Autodesk Inventor part; units mm, degrees
ref_plane "YZ Plane" through (0, 0, 0) normal (1, 0, 0) x (0, 1, 0)
ref_plane "XZ Plane" through (0, 0, 0) normal (0, 1, 0) x (-1, 0, 0)
ref_plane "XY Plane" through (0, 0, 0) normal (0, 0, 1) x (1, 0, 0)
sketch "スケッチ1" plane through (0, 0, 0) normal (0, 0, 1) x (1, 0, 0)
  line L0 (0, 31) -> (26, 31)
  line L1 (26, 31) -> (26, 0)
  line L2 (26, 0) -> (0, 0)
  line L3 (0, 0) -> (0, 31)
  circle A0 centre (13, 31) radius 27.5
  point P0 (26, 6.7668)
  point P1 (0, 6.7668)
  dimension "d0" = 55
  dimension "d1" = 31
  dimension "d3" = 26
extrude "押し出し1" add sketch "スケッチ1" along normal blind 30 contours A0 L1 L2 L3
sketch "スケッチ2" plane through (0, 0, 0) normal (0, -1, 0) x (1, 0, 0)
  line L0 (26, 0) -> (0, 30)
  line L1 (0, 0) -> (26, 30)
  line L2 (22, 4.6154) -> (4, 4.6154)
  line L3 (4, 4.6154) -> (4, 25.3846)
  line L4 (4, 25.3846) -> (22, 25.3846)
  line L5 (22, 25.3846) -> (22, 4.6154)
  line L6 (26, 0) -> (26, 30)
  line L7 (26, 0) -> (0, 0)
  line L8 (0, 0) -> (0, 32)
  circle A0 centre (22, 4.6154) radius 0.8
  circle A1 centre (4, 4.6154) radius 0.8
  circle A2 centre (4, 25.3846) radius 0.8
  circle A3 centre (22, 25.3846) radius 0.8
  dimension "d6" = 4
  dimension "d7" = 1.6
  dimension "d8" = 1.6
  dimension "d9" = 1.6
  dimension "d10" = 1.6
extrude "押し出し2" cut sketch "スケッチ2" against normal through all contours A0 L2 L0 | L0 L5 A0 | L2 A0 L0 | L0 A0 L5 | A3 L5 L1 | L1 L4 A3 | A1 L3 L1 | L1 L2 A1 | L2 L1 A1 | L5 A3 L1 | L1 A3 L4 | L3 A1 L1 | A2 L4 L0 | L0 L3 A2 | A2 L0 L4 | L3 L0 A2
properties part number "toe_back_buf"
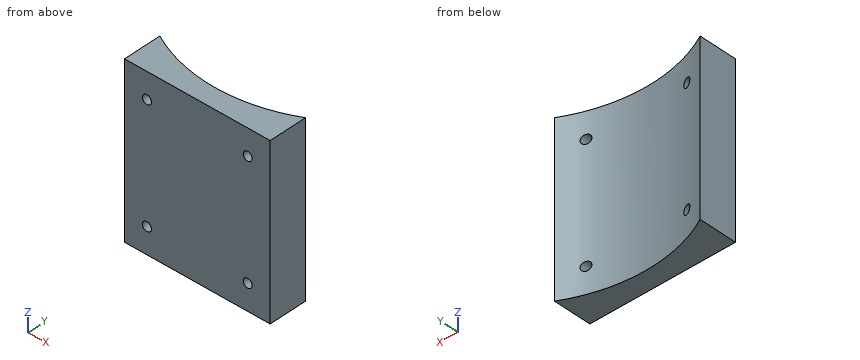
Geometry: final body of the model. Coordinates: model frame, mm. Round coordinates to 2 decimals unless told otherwise and drop trailing zeros. Order: outer loops, then holes, each group sorted by start corner. A loop starts at its lowest first (then second) coordinate and runs counter-clockwise, first axis right, second up. Notation, with made-up numbers: (-4, 58.5) - (33, 58.5) arc R10 cw to (33, 76.5) - close; hole circle Ø2 at (76.5, -19). An arc over 180 degrees is marked (long way). Write each question's results on one line, items separated by ' | '.
Item 1: Material intervals for line 1 along Z through (x, y) = (4, 4.05); line 2 along X through (y, z) = (2, 25); line 3 along X through (y, z) = (1.25, 4), sorted ascending. Write a range as [from, to].
Completed:
line 1: [0, 3.82], [5.42, 24.58], [26.18, 30] | line 2: [0, 3.3], [4.7, 21.3], [22.7, 26] | line 3: [0, 3.49], [4.51, 21.49], [22.51, 26]
Item 2: Section D-D, the plane x = 7.25. Return the cut outline in (y, z).
Completed:
outline: (0, 0) - (4.11, 0) - (4.11, 30) - (0, 30) - close
Item 3: Section B-B, the plane x = 4. Return the cut outline in (y, z), and give its area (3 significant figures).
Completed:
outline: (0, 0) - (5.01, 0) - (5.01, 3.82) - (0, 3.82) - close; (0, 5.42) - (5.01, 5.42) - (5.01, 24.58) - (0, 24.58) - close; (0, 26.18) - (5.01, 26.18) - (5.01, 30) - (0, 30) - close | area: 134 mm^2
Item 4: Section A-A, the plane y = 4. Return the cut outline in (x, z).
Completed:
outline: (0, 0) - (7.78, 0) - (7.78, 30) - (0, 30) - close; (18.22, 0) - (26, 0) - (26, 30) - (18.22, 30) - close; hole circle Ø1.6 at (4, 4.62); hole circle Ø1.6 at (4, 25.38); hole circle Ø1.6 at (22, 4.62); hole circle Ø1.6 at (22, 25.38)
Item 5: First-contact query: pin 1 Ø2 at (x, z) = (4, 25.38) entering from +Y; pin 2 Ø1.4 at (x, z) = (22, 4.62) entering from +Y; pin 3 Ø3 at (x, z) = (7.5, 8) entering from +Y; pin 4 Ø6 at (x, z) = (11.5, 20) entering from +Y. Flat tips, straight axial feed; report the tip coordinate or a pass-through.
Completed:
pin 1: y = 5.38 | pin 2: through | pin 3: y = 4.41 | pin 4: y = 3.87
Item 6: Section C-C, the plane z = 11. Return the cut outline in (x, y).
Completed:
outline: (0, 0) - (26, 0) - (26, 6.77) arc R27.5 cw to (0, 6.77) - close
